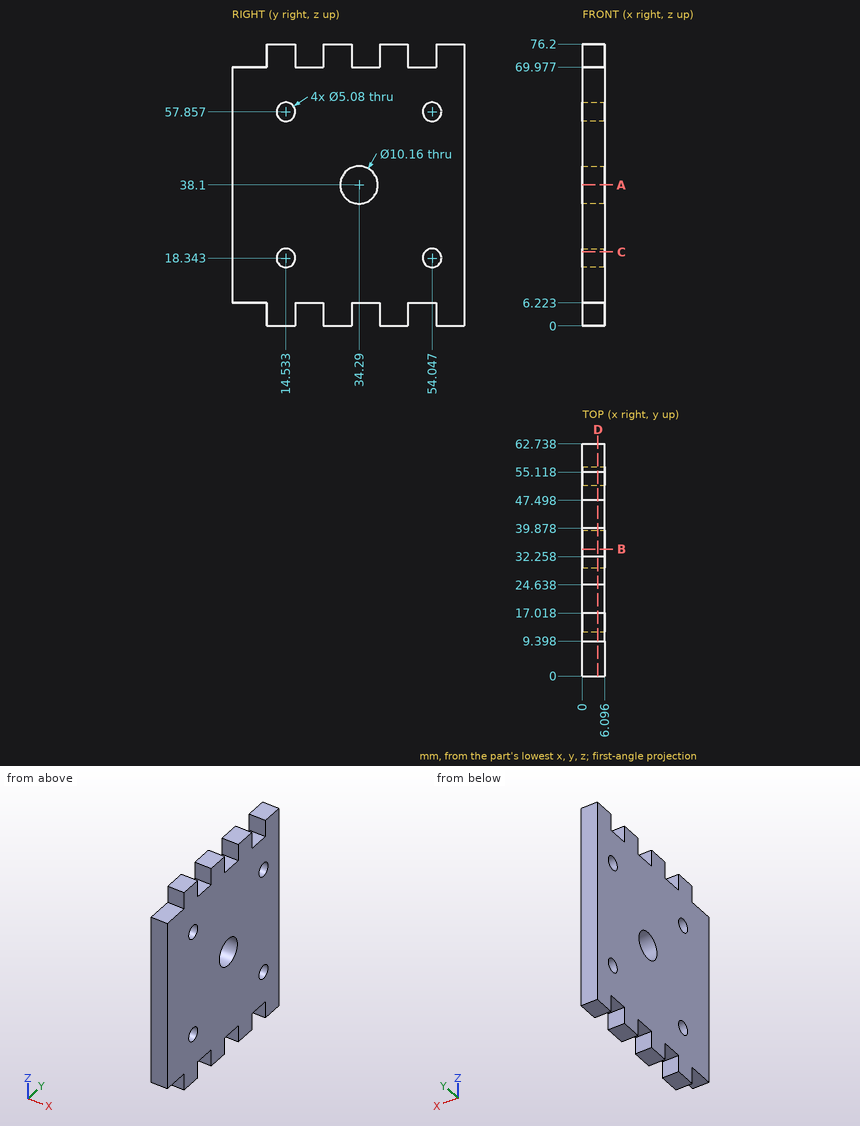
Study the drawing (mm; zero at the part's minimum x, y, z) and answer. Round coordinates to 2 decimals unless told otherwise and drop trailing zeros. Write each loop counter-clockwise with the first axis right and the second up, starting at its lowest first coordinate (ties: lowest second). Pieces come first, ordered by that corner, then holes. Notation, with made-up numbers: (70.25, 58.25) - (102.25, 58.25) arc R26 ccw to (102.25, 92.25) - close; hole circle Ø10 at (73.25, 22). An arc over 180 degrees is marked (long way). Return JSON: item names as keys, results as strings. Group by question number.
Q1. Each of these flat-tipped pins is pushed along its axis until it touches: pin 1 Ø4 at (y, z) = (54.05, 57.86) entering from -X; pin 2 Ø1.8 at (x, y) = (3, 52.5) entering from -Z; pin 3 Ø1.8 at (x, y) = (2.5, 51) entering from +Z. Where does it stop, or does it pass through?
Q2. Find the intervals of material crossed by L1, parallel to Y at x = 1.75, z = 73; L2, parallel to Z at x = 4.25, y = 54; L3, parallel to Z at x = 4, y = 55, in increasing order.
Q3. The part is cut by section A-A on z = 38.1. Write down the section's boundary in (x, y).
Q4. The part is cut by section C-C on z = 20. Write down the section's boundary in (x, y).
Q5. The part is cut by section B-B on y = 34.29. Write down the section's boundary in (x, z), then the cut area to 3 significant figures.
Q6. The part is cut by section D-D on x = 4.25. Count the separate pieces of the cut face and the enclosed holes in it, then the cut area to 3 significant figures.
Solved:
{
 "1": {"pin 1": "through", "pin 2": "z = 6.22", "pin 3": "z = 69.98"},
 "2": {"L1": "9.4 to 17.02, 24.64 to 32.26, 39.88 to 47.5, 55.12 to 62.74", "L2": "6.22 to 15.8, 20.88 to 55.32, 60.4 to 69.98", "L3": "6.22 to 15.99, 20.7 to 55.5, 60.21 to 69.98"},
 "3": {"outline": "(0, 0) - (6.1, 0) - (6.1, 29.21) - (0, 29.21) - close; (0, 39.37) - (6.1, 39.37) - (6.1, 62.74) - (0, 62.74) - close"},
 "4": {"outline": "(0, 0) - (6.1, 0) - (6.1, 12.61) - (0, 12.61) - close; (0, 16.46) - (6.1, 16.46) - (6.1, 52.12) - (0, 52.12) - close; (0, 55.97) - (6.1, 55.97) - (6.1, 62.74) - (0, 62.74) - close"},
 "5": {"outline": "(0, 6.22) - (6.1, 6.22) - (6.1, 33.02) - (0, 33.02) - close; (0, 43.18) - (6.1, 43.18) - (6.1, 69.98) - (0, 69.98) - close", "area": "327 mm²"},
 "6": {"separate pieces": "1", "enclosed holes": "5", "area": "4,220 mm²"}
}
